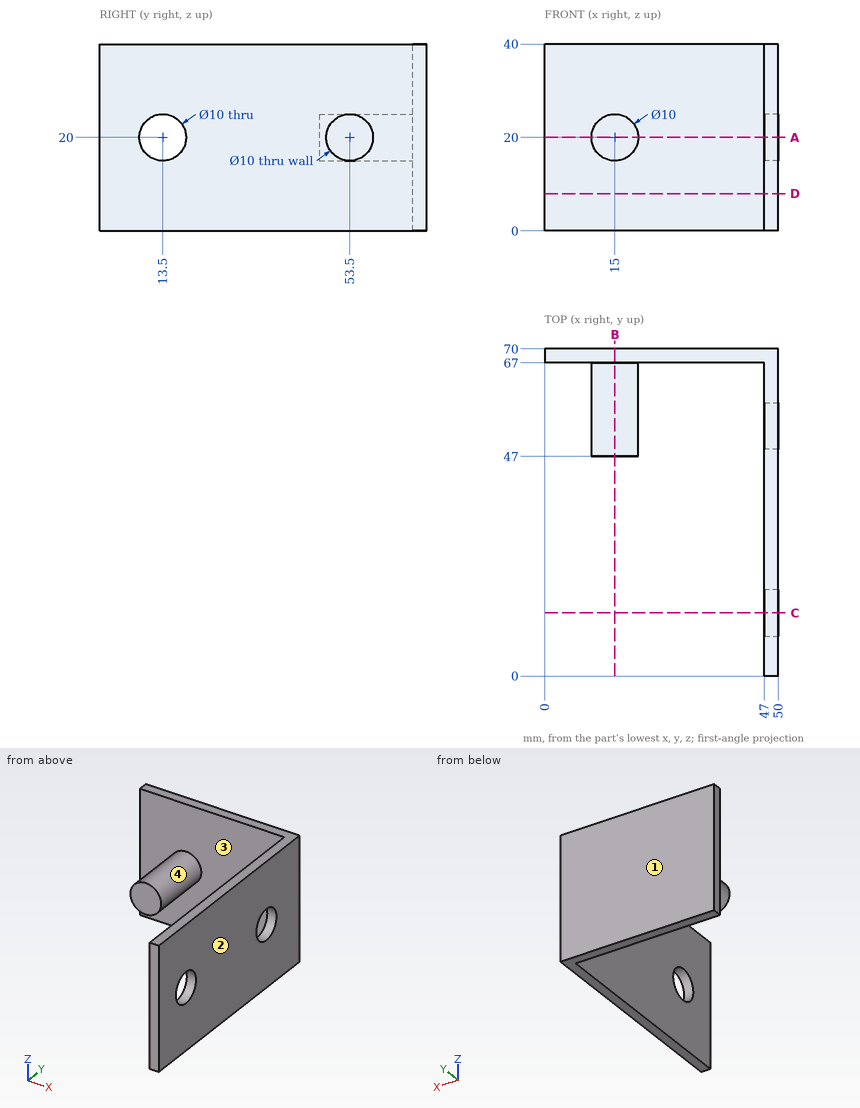
The figure shows three views and two pictorial views of one solid part (mm, origin at its lowest corner). Answer the questions. Give positions to 0.01 mm unless a question says otherwise; leave off trailing zeros. Order: outer loops, then holes, each group sorted by start corner. A loop starts at its lowest first (then second) coordinate and runs counter-clockwise, first axis right, second up. Notation, with made-up numbers: (14.5, 29.5) -> (53.5, 29.5) arc R24 cw to (53.5, 44.5) -> close; hole circle Ø9 at (38, -1.5). An arc over 180 degrees is marked (long way). Answer as CSV lines item,"result". Start each with the question number.
(1) For a pull along X with two mould halves and no side action, classify the marked faces 1, 2, 3 and 4 as released by +X, released by -X, zero draft, split by the parting line, or undercut.
(2) Section D-D, the plane z = 8 is taken. Write down the section's boundary in (x, y).
(3) Section A-A, the plane z = 20 is taken. Write down the section's boundary in (x, y).
(4) Each of these flat-tipped pins is pushed along its axis until it touches: pin 1 Ø8 at (y, z) = (38.5, 25.5) entering from -X; pin 2 Ø1.5 at (x, z) = (27, 32) entering from -Y; pin 3 Ø11 at (x, z) = (13, 21) entering from -Y. Where does it stop, or does it pass through?
(5) Section B-B, the plane x = 15 is taken. Write down the section's boundary in (y, z), plus the area to 3 significant figures.
(6) Section C-C, the plane y = 13.5 is taken. Write down the section's boundary in (x, z).
(7) Consider line 1 along Z through (x, y) = (47.9, 13.5); line 2 along Y through (x, z) = (17, 31); line 3 along X through (y, z) = (50, 4.5). Determine where each line is inside the solid, lowest interval first.
Entries:
1,face 1,"zero draft"
1,face 2,"released by +X"
1,face 3,"undercut"
1,face 4,"undercut"
2,outline,"(0, 67) -> (47, 67) -> (47, 0) -> (50, 0) -> (50, 70) -> (0, 70) -> close"
3,outline,"(0, 67) -> (10, 67) -> (10, 47) -> (20, 47) -> (20, 67) -> (47, 67) -> (47, 58.5) -> (50, 58.5) -> (50, 70) -> (0, 70) -> close; (47, 0) -> (50, 0) -> (50, 8.5) -> (47, 8.5) -> close; (47, 18.5) -> (50, 18.5) -> (50, 48.5) -> (47, 48.5) -> close"
4,pin 1,"x = 47"
4,pin 2,"y = 67"
4,pin 3,"y = 47"
5,outline,"(47, 15) -> (67, 15) -> (67, 0) -> (70, 0) -> (70, 40) -> (67, 40) -> (67, 25) -> (47, 25) -> close"
5,area,"320 mm²"
6,outline,"(47, 0) -> (50, 0) -> (50, 15) -> (47, 15) -> close; (47, 25) -> (50, 25) -> (50, 40) -> (47, 40) -> close"
7,line 1,"0 to 15, 25 to 40"
7,line 2,"67 to 70"
7,line 3,"47 to 50"
